For this review, take the finished solid that the model builds, in its own axes (mm). Face numbers are marked on the shaded views. A direction names the side the tool comes from. Round coordinates to 2 decimals unless told otherwise and drop trailing zeros. Write each loop counter-clockwise with the first axis right and the second up, starting at its lowest first coordinate (ties: lowest second). Pieces come first, ordered by that corner, then holes. Notation, with made-up numbers: M 18.25,-21.5 L 30.25,-21.5 A14 cw 30.25,-9.5 Z; hole C 4.5,23.5 d6. An arc over 180 degrees is marked long. Use one line per item in the form item = value. Start each with the question number.
Item 1: Draft analysis for pull direction Y (two halves, no side actions). For the marked faces 1, 2, 3 and 4, state which applies: released by +Y, released by -Y, zero draft, split by the parting line, or undercut.
Item 2: Add section B-B (x = 0). State the section outline as (y, z) points, and give its area (3 significant figures).
Item 3: Add section A-A (z = -13). State the section outline as (x, y) points, and give its area (3 significant figures).
Item 4: For P1, Ø11.5, axis at x = 3.5, y = 19, coming from the -Z side; P2, Ø2, axis at x = -11.5, y = 1, coming from the +Z side; P3, Ø1, axis at x = -6.5, y = 40.5, coming from the -Z side, all flat-tipped, find the tip position at first contact; note any pin that passes through.
Item 5: For the marked faces 5, 6, 7 and 8, list the 3-axis set-ups (+Z, -Z, +X, -X, +Y, -Y) from which the entire face can be reached by the end or side of a thin tool; tool diameter is ignored.
Item 6: For line 1 (X direction, y = 40.5, z = 23.75); line 2 (Y direction, x = 10, z = 10); line 3 (Y direction, x = 14, z = 24), list the stretches that pass through material, from the lowest coordinate up. Write a range as [from, to].
Item 7: Add section C-C (x = -10.5). State the section outline as (y, z) points, and give its area (3 significant figures).
Item 8: Add section D-D (y = 17). State the section outline as (x, z) points, and give its area (3 significant figures).
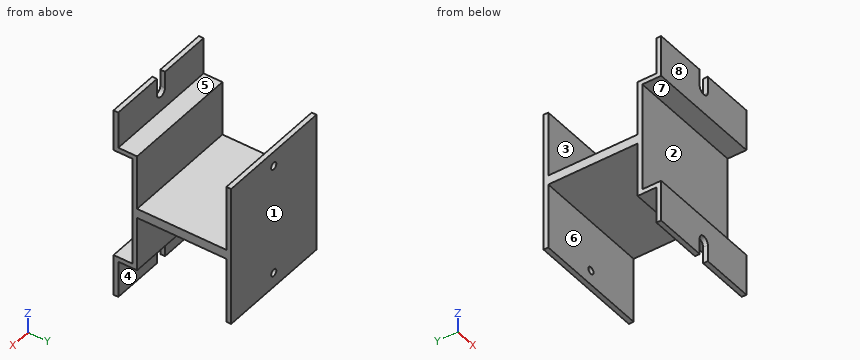
from build123d import *

# Parameters (mm, degrees)
EXTRUDE_THIN1_DEPTH = 25
EXTRUDE_THIN2_DEPTH = 25
CUT_EXTRUDE1_DEPTH  = 10
SKETCH4_R           = 1.5
CUT_EXTRUDE2_DEPTH  = 3


with BuildPart() as part:
    # Sketch1 → Extrude-Thin1 (new, symmetric)
    with BuildSketch(Plane(origin=(0, 0, 0), x_dir=(0, 0, -1), z_dir=(1, 0, 0))):
        Polygon((0, 0), (23.333492345, 0), (23.333492345, -8), (41, -8), (41, -6), (25.333492345, -6), (25.333492345, 2), (0, 2), align=None)
    extrude(amount=EXTRUDE_THIN1_DEPTH, both=True)

    # Sketch2 → Extrude-Thin2 (add, symmetric)
    with BuildSketch(Plane(origin=(0, 0, 0), x_dir=(0, 0, -1), z_dir=(1, 0, 0))):
        Polygon((0, 0), (0, 42), (30, 42), (30, 40), (2, 40), (2, 0), align=None)
    extrude(amount=EXTRUDE_THIN2_DEPTH, both=True)

    # Mirror1: part across face


with BuildPart() as part_1:
    add(part.part)
    add(part.part.mirror(Plane(origin=(0, 21, 0), x_dir=(1, 0, 0), z_dir=(0, 0, 1))))

    # Sketch3 → Cut-Extrude1 (cut)
    with BuildSketch(Plane(origin=(0, -6, 0), x_dir=(1, 0, 0), z_dir=(0, 1, 0))):
        with BuildLine():
            Line((-2.375, 33.875), (-2.375, 51.560435524))
            ThreePointArc((-2.375, 51.560435524), (0, 53.935435524), (2.375, 51.560435524))
            Line((2.375, 51.560435524), (2.375, 33.875))
            ThreePointArc((2.375, 33.875), (0, 31.5), (-2.375, 33.875))
        make_face()
        with BuildLine():
            Line((-2.375, -33.875), (-2.375, -51.560435524))
            ThreePointArc((-2.375, -51.560435524), (0, -53.935435524), (2.375, -51.560435524))
            Line((2.375, -51.560435524), (2.375, -33.875))
            ThreePointArc((2.375, -33.875), (0, -31.5), (-2.375, -33.875))
        make_face()
    extrude(amount=-CUT_EXTRUDE1_DEPTH, mode=Mode.SUBTRACT)

    # Sketch4 → Cut-Extrude2 (cut)
    with BuildSketch(Plane(origin=(0, 42, 0), x_dir=(1, 0, 0), z_dir=(0, 1, 0))):
        with Locations(Location((0, 23.75, 0), (0, 0, 270))):
            Circle(SKETCH4_R)
        with Locations(Location((0, -23.75, 0), (0, 0, 270))):
            Circle(SKETCH4_R)
    extrude(amount=-CUT_EXTRUDE2_DEPTH, mode=Mode.SUBTRACT)


solid = part_1.part
Calculated:
q1.face_1 = released by +Y
q1.face_2 = released by -Y
q1.face_3 = undercut
q1.face_4 = undercut
q2.outline = M -8,-31.5 L -6,-31.5 L -6,-25.33 L 2,-25.33 L 2,-2 L 40,-2 L 40,-22.25 L 42,-22.25 L 42,22.25 L 40,22.25 L 40,2 L 2,2 L 2,25.33 L -6,25.33 L -6,31.5 L -8,31.5 L -8,23.33 L 0,23.33 L 0,-23.33 L -8,-23.33 Z; M 40,-30 L 42,-30 L 42,-25.25 L 40,-25.25 Z; M 40,25.25 L 42,25.25 L 42,30 L 40,30 Z
q2.area = 418 mm^2
q3.outline = M -25,0 L 25,0 L 25,2 L -25,2 Z; M -25,40 L 25,40 L 25,42 L -25,42 Z
q3.area = 200 mm^2
q4.P1 = -2
q4.P2 = 25.33
q4.P3 = -30
q5.face_5 = +Z, +X, -X
q5.face_6 = -Z, +X, -X
q5.face_7 = +X, -X, -Y
q5.face_8 = +Z, -Z, +X, -X, -Y
q6.line_1 = [-25, -1.5], [1.5, 25]
q6.line_2 = [0, 2], [40, 42]
q6.line_3 = [-8, 2], [40, 42]
q7.outline = M -8,-41 L -6,-41 L -6,-25.33 L 2,-25.33 L 2,-2 L 40,-2 L 40,-30 L 42,-30 L 42,30 L 40,30 L 40,2 L 2,2 L 2,25.33 L -6,25.33 L -6,41 L -8,41 L -8,23.33 L 0,23.33 L 0,-23.33 L -8,-23.33 Z
q7.area = 468 mm^2
q8.outline = M -25,-2 L 25,-2 L 25,2 L -25,2 Z
q8.area = 200 mm^2
